```python
from build123d import *

# Parameters (mm, degrees)
ESQUISSE1_W      = 241
ESQUISSE1_H      = 48
ESQUISSE1_R      = 2
EXTRUSION1_DEPTH = 12.5
ESQUISSE2_W      = 9
ESQUISSE2_H      = 11
EXTRUSION2_DEPTH = 49
EXTRUSION3_REACH = 50
ESQUISSE3_R      = 3


with BuildPart() as part:
    # Esquisse1 → Extrusion1 (new body)
    with BuildSketch(Plane.XY):
        with Locations((120.5, -24)):
            Rectangle(ESQUISSE1_W, ESQUISSE1_H)
        with Locations((195, -39)):
            Circle(ESQUISSE1_R, mode=Mode.SUBTRACT)
        with Locations((46, -9)):
            Circle(ESQUISSE1_R, mode=Mode.SUBTRACT)
        with Locations((46, -39)):
            Circle(ESQUISSE1_R, mode=Mode.SUBTRACT)
        with Locations((195, -9)):
            Circle(ESQUISSE1_R, mode=Mode.SUBTRACT)
    extrude(amount=EXTRUSION1_DEPTH)

    # Esquisse2 → Extrusion2 (cut, through all)
    with BuildSketch(Plane(origin=(0, 0, 0), x_dir=(1, 0, 0), z_dir=(0, 1, 0))):
        with Locations((4.5, -5.5)):
            Rectangle(ESQUISSE2_W, ESQUISSE2_H)
        with Locations((236.5, -5.5)):
            Rectangle(ESQUISSE2_W, ESQUISSE2_H)
    extrude(amount=-EXTRUSION2_DEPTH, mode=Mode.SUBTRACT)

    # Esquisse3 → Extrusion3 (cut, up to next)
    with BuildSketch(Plane(origin=(0, 0, 0), x_dir=(1, 0, 0), z_dir=(0, 1, 0)), mode=Mode.PRIVATE) as extrusion3_sk1:
        with Locations((120.5, -6.25)):
            Circle(ESQUISSE3_R)
    extrusion3_tool1 = extrude(extrusion3_sk1.sketch, amount=-EXTRUSION3_REACH, mode=Mode.PRIVATE) & part.part
    add(extrusion3_tool1.solids().sort_by_distance((120.5, 0, 6.25))[0], mode=Mode.SUBTRACT)
    # Esquisse3 → Extrusion3 (cut, up to next)
    with BuildSketch(Plane(origin=(0, 0, 0), x_dir=(1, 0, 0), z_dir=(0, 1, 0)), mode=Mode.PRIVATE) as extrusion3_sk2:
        with Locations((24.5, -6.25)):
            Circle(ESQUISSE3_R)
    extrusion3_tool2 = extrude(extrusion3_sk2.sketch, amount=-EXTRUSION3_REACH, mode=Mode.PRIVATE) & part.part
    add(extrusion3_tool2.solids().sort_by_distance((24.5, 0, 6.25))[0], mode=Mode.SUBTRACT)
    # Esquisse3 → Extrusion3 (cut, up to next)
    with BuildSketch(Plane(origin=(0, 0, 0), x_dir=(1, 0, 0), z_dir=(0, 1, 0)), mode=Mode.PRIVATE) as extrusion3_sk3:
        with Locations((216.5, -6.25)):
            Circle(ESQUISSE3_R)
    extrusion3_tool3 = extrude(extrusion3_sk3.sketch, amount=-EXTRUSION3_REACH, mode=Mode.PRIVATE) & part.part
    add(extrusion3_tool3.solids().sort_by_distance((216.5, 0, 6.25))[0], mode=Mode.SUBTRACT)


solid = part.part
```
Part model, mm, in its own coordinate system. A direction names the side the tool comes from. Coordinates: 2 decimals unless noted, no trailing zeros. Write each loop counter-clockwise with the first axis right and the second up, starting at its lowest first coordinate (ties: lowest second). Pieces come first, ordered by that corner, then holes.
Item 1: Mould opens along Z. For faces 1 (the face through (4, -24, 11)), 2 (the face through (193, -9, 6)), 3 (the face through (22.29, -23.66, 4.22)) say: released by +Z, released by -Z, zero draft, split by the parting line, or undercut.
Item 2: Which spindle directions (+Z, -Z, +X, -X, +Y, -Y) get a long thin tool onto all of the face, cutting with end or side? Do faces 4 (the face through (236, -24, 11)), 5 (the face through (119, -24, 12.5)), 6 (the face through (9, -24, 6)). Say none if no direction does.
Item 3: Pin check, flat tips, straight feed: pin 1 (1.5 mm diameter, centred on y = -41, z = 9, fed in from +X); pin 2 (5 mm diameter, centred on x = 120.5, z = 6.25, fed in from +Y); pin 3 (1.5 mm diameter, centred on y = -42, z = 3.5, fed in from -X); pin 4 (2.5 mm diameter, centred on x = 235.5, y = -34.5, fed in from -Z). Stop position of each tip, or through.
Item 4: Slice it at A-A (z = 6.25). Write the cut outline in (x, y), and give its area (3 significant figures).
Item 5: Probe line 1 (X direction, y = -21.5, z = 6); line 2 (Y direction, x = 195, z = 3.5); line 3 (Y direction, x = 193.5, z = 5.75). List the from-to ranges inside material, lowest first.
Item 6: Slice it at B-B (x = 46). Write the cut outline in (y, z), and give its area (3 significant figures).
Item 7: Slice it at D-D (x = 120.5). Write the cut outline in (y, z), and give its area (3 significant figures).
Item 8: Slice it at C-C (y = -39). Write the cut outline in (x, z).
Results found:
1. face 1: released by -Z
1. face 2: zero draft
1. face 3: undercut
2. face 4: -Z, +X, +Y, -Y
2. face 5: +Z, +X, -X, +Y, -Y
2. face 6: -Z, -X, +Y, -Y
3. pin 1: stops at x = 232
3. pin 2: passes through
3. pin 3: stops at x = 9
3. pin 4: stops at z = 11
4. outline: (9, -48) - (21.5, -48) - (21.5, 0) - (9, 0) - close; (27.5, -48) - (117.5, -48) - (117.5, 0) - (27.5, 0) - close; (123.5, -48) - (213.5, -48) - (213.5, 0) - (123.5, 0) - close; (219.5, -48) - (232, -48) - (232, 0) - (219.5, 0) - close; hole circle Ø4 at (46, -39); hole circle Ø4 at (46, -9); hole circle Ø4 at (195, -39); hole circle Ø4 at (195, -9)
4. area: 9,790 mm2
5. line 1: x = 9 to 21.51, 27.49 to 117.51, 123.49 to 213.51, 219.49 to 232
5. line 2: y = -48 to -41, -37 to -11, -7 to 0
5. line 3: y = -48 to -40.32, -37.68 to -10.32, -7.68 to 0
6. outline: (-48, 0) - (-41, 0) - (-41, 12.5) - (-48, 12.5) - close; (-37, 0) - (-11, 0) - (-11, 12.5) - (-37, 12.5) - close; (-7, 0) - (0, 0) - (0, 12.5) - (-7, 12.5) - close
6. area: 500 mm2
7. outline: (-48, 0) - (0, 0) - (0, 3.25) - (-48, 3.25) - close; (-48, 9.25) - (0, 9.25) - (0, 12.5) - (-48, 12.5) - close
7. area: 312 mm2
8. outline: (0, 11) - (9, 11) - (9, 0) - (44, 0) - (44, 12.5) - (0, 12.5) - close; (48, 0) - (193, 0) - (193, 12.5) - (48, 12.5) - close; (197, 0) - (232, 0) - (232, 11) - (241, 11) - (241, 12.5) - (197, 12.5) - close; hole circle Ø6 at (24.5, 6.25); hole circle Ø6 at (120.5, 6.25); hole circle Ø6 at (216.5, 6.25)
